Read the model definition and answer for the solid it produces. Units are mm, in the model's axes. Face numbers are marked on the shaded views. A direction names the side the tool comes from. Give positions to 0.01 mm unless a question says otherwise; leave off trailing zeros. Order: outer loops, then holes, each group sorted by start corner. A loop starts at its lowest first (then second) coordinate and runs counter-clockwise, first axis right, second up.
```python
from build123d import *

# Parameters (mm, degrees)
SKETCH1_R           = 20.5
SKETCH1_R_2         = 1.6
SKETCH1_R_3         = 5
BOSS_EXTRUDE1_DEPTH = 20
SKETCH2_W           = 60
SKETCH2_H           = 80
SKETCH2_R           = 20.5
BOSS_EXTRUDE2_DEPTH = 10
CUT_EXTRUDE1_DEPTH  = 5
FILLET1_R           = 10
SKETCH4_R           = 5
CUT_EXTRUDE2_DEPTH  = 7


with BuildPart() as part:
    # Sketch1 → Boss-Extrude1 (new body)
    with BuildSketch(Plane(origin=(0, 0, 0), x_dir=(1, 0, 0), z_dir=(0, 1, 0))):
        with Locations(Location((0, 0, 0), (0, 0, 270))):
            Circle(SKETCH1_R)
        with Locations(Location((6.314276634, 15.244012286, 0), (0, 0, 270))):
            Circle(SKETCH1_R_2, mode=Mode.SUBTRACT)
        with Locations(Location((10.044563579, -13.090330115, 0), (0, 0, 270))):
            Circle(SKETCH1_R_2, mode=Mode.SUBTRACT)
        with Locations(Location((-16.358840213, -2.153682172, 0), (0, 0, 270))):
            Circle(SKETCH1_R_2, mode=Mode.SUBTRACT)
        with Locations(Location((0, 0, 0), (0, 0, 270))):
            Circle(SKETCH1_R_3, mode=Mode.SUBTRACT)
    extrude(amount=BOSS_EXTRUDE1_DEPTH)

    # Sketch2 → Boss-Extrude2 (add)
    with BuildSketch(Plane.XZ):
        Rectangle(SKETCH2_W, SKETCH2_H)
        with Locations(Location((0, 0, 0), (0, 0, 270))):
            Circle(SKETCH2_R, mode=Mode.SUBTRACT)
        with BuildLine():
            Line((-12.5, 34), (12.5, 34))
            ThreePointArc((12.5, 34), (16.5, 30), (12.5, 26))
            Line((12.5, 26), (-12.5, 26))
            ThreePointArc((-12.5, 26), (-16.5, 30), (-12.5, 34))
        make_face(mode=Mode.SUBTRACT)
        with BuildLine():
            Line((-12.5, -34), (12.5, -34))
            ThreePointArc((12.5, -34), (16.5, -30), (12.5, -26))
            Line((12.5, -26), (-12.5, -26))
            ThreePointArc((-12.5, -26), (-16.5, -30), (-12.5, -34))
        make_face(mode=Mode.SUBTRACT)
    extrude(amount=-BOSS_EXTRUDE2_DEPTH)

    # Sketch3 → Cut-Extrude1 (cut)
    with BuildSketch(Plane(origin=(0, 10, 0), x_dir=(1, 0, 0), z_dir=(0, 1, 0))):
        with BuildLine():
            Line((-12.5, 38.5), (12.5, 38.5))
            ThreePointArc((12.5, 38.5), (21, 30), (12.5, 21.5))
            Line((12.5, 21.5), (-12.5, 21.5))
            ThreePointArc((-12.5, 21.5), (-21, 30), (-12.5, 38.5))
        make_face()
        with BuildLine():
            Line((-12.5, -38.5), (12.5, -38.5))
            ThreePointArc((12.5, -38.5), (21, -30), (12.5, -21.5))
            Line((12.5, -21.5), (-12.5, -21.5))
            ThreePointArc((-12.5, -21.5), (-21, -30), (-12.5, -38.5))
        make_face()
    extrude(amount=-CUT_EXTRUDE1_DEPTH, mode=Mode.SUBTRACT)

    # Fillet1
    fillet1_edges = [part.edges().sort_by_distance(p)[0] for p in [
        (30, 5, 40),
        (30, 5, -40),
        (-30, 5, -40),
        (-30, 5, 40),
    ]]
    fillet(fillet1_edges, radius=FILLET1_R)

    # Sketch4 → Cut-Extrude2 (cut)
    with BuildSketch(Plane.XZ):
        with Locations(Location((10.044563579, 13.090330115, 0), (0, 0, 270))):
            Circle(SKETCH4_R)
        with Locations(Location((6.314276634, -15.244012286, 0), (0, 0, 270))):
            Circle(SKETCH4_R)
        with Locations(Location((-16.358840213, 2.153682172, 0), (0, 0, 270))):
            Circle(SKETCH4_R)
    extrude(amount=-CUT_EXTRUDE2_DEPTH, mode=Mode.SUBTRACT)


solid = part.part
```
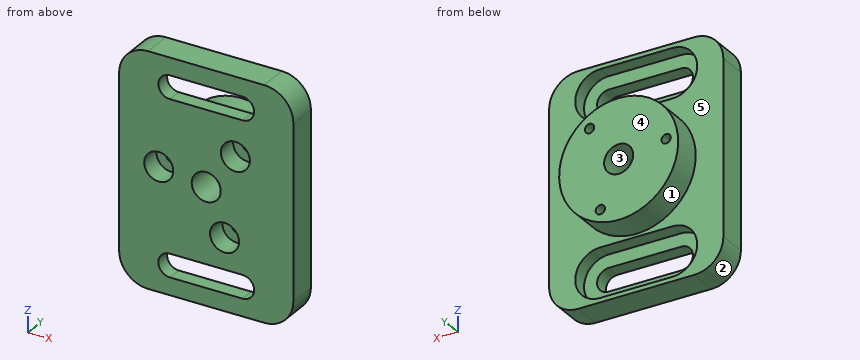
1) Given pin 1 (13.5 mm diameter, centred on x = 8.5, z = 30, fed in from +Y); pin 2 (5 mm diameter, centred on x = -16.36, z = 2.15, fed in from -Y); pin 3 (1.9 mm diameter, centred on x = 10.04, z = 13.09, fed in from -Y); pin 4 (8 mm diameter, centred on y = 16, z = 11, fed in from +X), each flat-ended and moving along its own axis, determine where each tip first touches the part or whether it passes through.
Final values:
pin 1: stops at y = 5
pin 2: stops at y = 7
pin 3: passes through
pin 4: stops at x = 19.27
2) The part is cut by section C-C on y = 2.25. Determine the outline of the cut face in (x, z).
Final values:
outline: (-30, -30) arc R10 ccw to (-20, -40) - (20, -40) arc R10 ccw to (30, -30) - (30, 30) arc R10 ccw to (20, 40) - (-20, 40) arc R10 ccw to (-30, 30) - close; hole circle Ø10 at (-16.36, 2.15); hole (-12.5, -34) - (12.5, -34) arc R4 ccw to (12.5, -26) - (-12.5, -26) arc R4 ccw to start; hole (-12.5, 26) - (12.5, 26) arc R4 ccw to (12.5, 34) - (-12.5, 34) arc R4 ccw to start; hole circle Ø10 at (0, 0); hole circle Ø10 at (6.31, -15.24); hole circle Ø10 at (10.04, 13.09)
3) For a pull along X with two mould halves and no side action, classify the marked faces 1, 2 and 3 as released by +X, released by -X, zero draft, split by the parting line, or undercut.
Final values:
face 1: split by the parting line
face 2: released by -X
face 3: undercut
4) A tool of negligible diameter and unlimited length cuts with its end or side. For the marked faces 4 and 5, from which of +Z, -Z, +X, -X, +Y, -Y can it reach the whole face along a straight path? Write none if from no direction.
Final values:
face 4: +Z, -Z, +X, -X, +Y
face 5: +Y
5) The part is cut by section A-A on x = 0. Determine the outline of the cut face in (y, z), and give its area (3 significant figures).
Final values:
outline: (0, -40) - (10, -40) - (10, -38.5) - (5, -38.5) - (5, -34) - (0, -34) - close; (0, -26) - (5, -26) - (5, -21.5) - (10, -21.5) - (10, -20.5) - (20, -20.5) - (20, -5) - (0, -5) - close; (0, 5) - (20, 5) - (20, 20.5) - (10, 20.5) - (10, 21.5) - (5, 21.5) - (5, 26) - (0, 26) - close; (0, 34) - (5, 34) - (5, 38.5) - (10, 38.5) - (10, 40) - (0, 40) - close
area: 760 mm2
6) The part is cut by section B-B on z = -16. Determine the outline of the cut face in (x, y), and give its area (3 significant figures).
Final values:
outline: (-30, 0) - (1.37, 0) - (1.37, 7) - (4.9, 7) - (4.9, 20) - (-12.82, 20) - (-12.82, 10) - (-30, 10) - close; (7.72, 7) - (11.26, 7) - (11.26, 0) - (30, 0) - (30, 10) - (12.82, 10) - (12.82, 20) - (7.72, 20) - close
area: 750 mm2
7) Consider L1, parallel to X at y = 9.75, z = -29.5; L2, parallel to Z at x = -15.5, y = 7.25; L3, parallel to X at y = 4.25, z = 3. Determine where each line is inside the solid, lowest interval first.
Final values:
L1: x = -30 to -20.99, 20.99 to 30
L2: z = -40 to -37.95, -22.05 to 0.8, 3.5 to 22.05, 37.95 to 40
L3: x = -30 to -21.29, -11.43 to -4, 4 to 30
8) The part is cut by section D-D on y = 18.5. Determine the outline of the cut face in (x, z).
Final values:
outline: circle Ø41 at (0, 0); hole circle Ø3.2 at (-16.36, 2.15); hole circle Ø10 at (0, 0); hole circle Ø3.2 at (6.31, -15.24); hole circle Ø3.2 at (10.04, 13.09)
